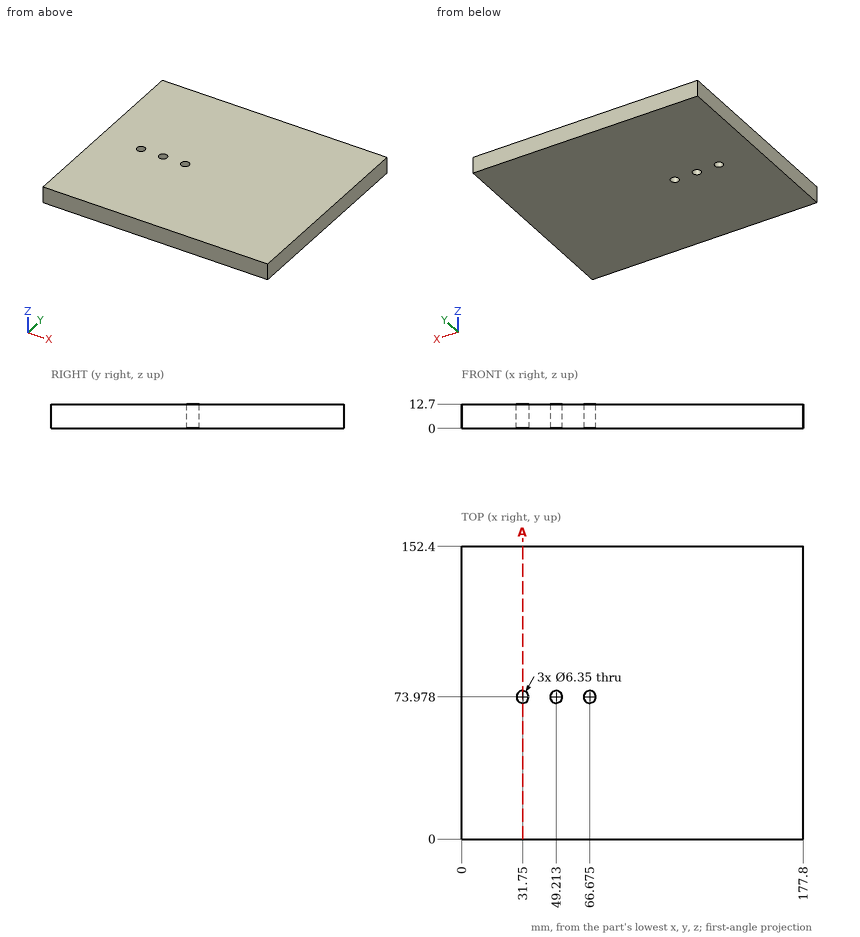
Geometry check sheet. Reference: drawing and pictorial views, mm from the part's lowest x, y, z. Give positions to 0.01 mm unless a question says otherwise; leave off trailing zeros. Order: outer loops, then holes, each group sorted by start corner. A loop starts at its lowest first (then second) coordinate and runs counter-clockwise, first axis right, second up. Notation, with made-up numbers: M -12,23 L 20,23 A25 cw 20,38 Z; hole C 33,80 d9. An arc over 180 degrees is marked long. Return JSON: item names as keys, results as strings. Group by question number.
1) Section check A-A on x = 31.75. Record the cut outline in (y, z).
2) Go/stop test with flat-tipped pins: pin 1 Ø10 at (x, y) = (75, 40.5) entering from -Z; pin 2 Ø5.5 at (x, y) = (66.68, 73.98) entering from +Z. Record where each tip stops, or that it passes through.
3) Scan lines: line 1 (Y direction, x = 31.75, z = 3.75); line 2 (Y direction, x = 69.5, z = 3.5) (1 decimal). Record each from-to range of solid material in increasing order.
Answer block:
{
 "1": {"outline": "M 0,0 L 70.8,0 L 70.8,12.7 L 0,12.7 Z; M 77.15,0 L 152.4,0 L 152.4,12.7 L 77.15,12.7 Z"},
 "2": {"pin 1": "stops at z = 0", "pin 2": "passes through"},
 "3": {"line 1": "y = 0 to 70.8, 77.15 to 152.4", "line 2": "y = 0 to 72.5, 75.4 to 152.4"}
}
